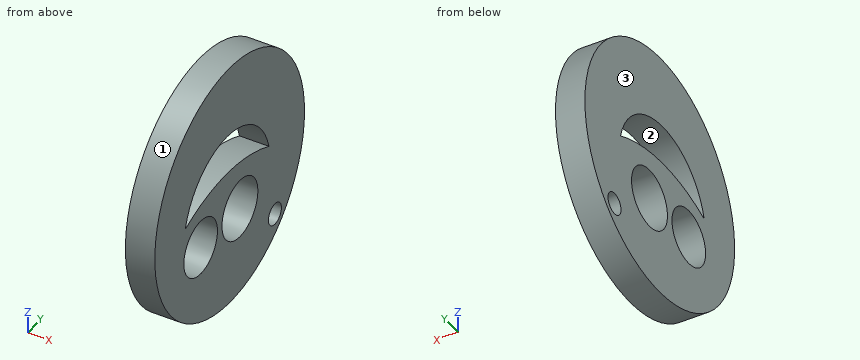
```python
from build123d import *

# Parameters (mm, degrees)
F0_R     = 21.58858
F1_DEPTH = 5.08
F2_R     = 4.849274
F2_R_2   = 5.175735
F3_DEPTH = 5.08
F4_R     = 1.874889
F5_DEPTH = 5.08


with BuildPart() as f1:
    # F0 (on Right) → F1 (new body)
    with BuildSketch(Plane.YZ):
        Circle(F0_R)
    extrude(amount=F1_DEPTH)

    # F2 (on face) → F3 (cut)
    with BuildSketch(Plane.YZ.offset(5.08)):
        with BuildLine():
            ThreePointArc((-12.801601, 0), (-0.738554, 2.638206), (11.324493, 0))
            ThreePointArc((11.324493, 0), (-0.738554, 9.394046), (-12.801601, 0))
        make_face()
        with Locations((-8.370277, -6.154616)):
            Circle(F2_R)
        with Locations((2.954216, -6.154616)):
            Circle(F2_R_2)
    extrude(amount=-F3_DEPTH, mode=Mode.SUBTRACT)

    # F4 (on face) → F5 (cut)
    with BuildSketch(Plane(origin=(0, 0, 0), x_dir=(0, -1, 0), z_dir=(-1, 0, 0))):
        with Locations((-13.047784, -13.540154)):
            Circle(F4_R)
    extrude(amount=-F5_DEPTH, mode=Mode.SUBTRACT)


solid = f1.part
```
Source: CAD feature listing. Evaluate the final solid. Frame: model axes, mm. Face numbers are marked on the shaded views. Give positions to 0.01 mm unless a question says otherwise; leave off trailing zeros. Loops run counter-clockwise (first coordinate to the right, second up) from the corner with the lowest first, then second, coordinate; pieces in that order, holes last. Notation, with made-up numbers: (-9, 41) - (12, 41) arc R13 ccw to (12, 57) - close; hole circle Ø11 at (12.25, 52). An arc over 180 degrees is marked (long way). Use CSV: the item, a comma, the result in double quotes.
1) Cut plane B-B (z = -4). Output: boundary loops of the cut face in (x, y), and give its area (3 significant figures).
Worked out:
outline,"(0, -21.21) - (5.08, -21.21) - (5.08, -12.71) - (0, -12.71) - close; (0, -4.03) - (5.08, -4.03) - (5.08, -1.75) - (0, -1.75) - close; (0, 7.66) - (5.08, 7.66) - (5.08, 21.21) - (0, 21.21) - close"
area,"124 mm^2"
2) Pin query (flat end, axial travel): P1, Ø1, axis at x = 2, z = 14, coming from the -Y side; P2, Ø1.5, axis at x = 1.5, z = 16.5, coming from the +Y side; P3, Ø1, axis at x = 2, y = 5, coming from the -Z side. Return the tip coordinate at first contact, or that it passes through.
Worked out:
P1,"stops at y = -16.85"
P2,"stops at y = 14.76"
P3,"stops at z = -21.11"
3) Line query: line 1 (Z direction, x = 3.45, y = -10.5); line 2 (Z direction, x = 4, y = -11.5); line 3 (Y direction, x = 3, z = 5.5). Output: solid intervals per line, ascending.
Worked out:
line 1,"z = -18.86 to -10.51, -1.8 to 0.94, 4.67 to 18.86"
line 2,"z = -18.27 to -9.86, -2.45 to 0.56, 3.2 to 18.27"
line 3,"y = -20.88 to -9.78, 8.3 to 20.88"
4) Cut plane D-D (y = -18). Output: boundary loops of the cut face in (x, z), and give its area (3 significant figures).
Worked out:
outline,"(0, -11.92) - (5.08, -11.92) - (5.08, 11.92) - (0, 11.92) - close"
area,"121 mm^2"
5) Mould query, pull axis Y, two halves, no side actions, for the marked faces 1, 2 and 3. Classes: +Y half, -Y half, draft (parallel to the pull), parting line (faces both ways), or undercut.
Worked out:
face 1,"parting line"
face 2,"undercut"
face 3,"draft"
6) Cut plane A-A (y = 0). Output: boundary loops of the cut face in (x, z).
Worked out:
outline,"(0, -21.59) - (5.08, -21.59) - (5.08, -10.4) - (0, -10.4) - close; (0, -1.9) - (5.08, -1.9) - (5.08, 2.63) - (0, 2.63) - close; (0, 9.37) - (5.08, 9.37) - (5.08, 21.59) - (0, 21.59) - close"
7) Cut plane C-C (x = 3.1). Output: boundary loops of the cut face in (y, z), and give its area (3 significant figures).
Worked out:
outline,"circle Ø43.18 at (0, 0); hole circle Ø9.7 at (-8.37, -6.15); hole (-12.8, 0) arc R28.9 cw to (11.32, 0) arc R12.44 ccw to start; hole circle Ø10.35 at (2.95, -6.15); hole circle Ø3.75 at (13.05, -13.54)"
area,"1,170 mm^2"
